```python
from build123d import *

# Parameters (mm, degrees)
BOX001_W         = 2
BOX001_H         = 37
BOX001_DEPTH     = 2
BOX_W            = 2
BOX_H            = 37
BOX_DEPTH        = 2
CIRCLE_R         = 1.75
EXTRUDE_DEPTH    = 2
CIRCLE001_R      = 1.75
EXTRUDE001_DEPTH = 2
CIRCLE002_R      = 1.75
EXTRUDE002_DEPTH = 2
CIRCLE003_R      = 1.75
EXTRUDE003_DEPTH = 2
RECTANGLE_W      = 43
RECTANGLE_H      = 43
EXTRUDE004_DEPTH = 2
FILLET_R         = 3
FILLET001_R      = 0.5
CHAMFER_SIZE     = 0.5
CHAMFER001_SIZE  = 0.5


with BuildPart() as cube001:
    # Box001 → Box001 (new body)
    with BuildSketch(Plane(origin=(30.5, 3, 0), x_dir=(1, 0, 0), z_dir=(0, 0, 1))):
        with Locations((1, 18.5)):
            Rectangle(BOX001_W, BOX001_H)
    extrude(amount=BOX001_DEPTH)


with BuildPart() as cube:
    # Box → Box (new body)
    with BuildSketch(Plane(origin=(10.5, 3, 0), x_dir=(1, 0, 0), z_dir=(0, 0, 1))):
        with Locations((1, 18.5)):
            Rectangle(BOX_W, BOX_H)
    extrude(amount=BOX_DEPTH)


with BuildPart() as extrude_body:
    # Circle → Extrude (new body)
    with BuildSketch(Plane(origin=(36.75, 6.25, 0), x_dir=(1, 0, 0), z_dir=(0, 0, 1))):
        Circle(CIRCLE_R)
    extrude(amount=EXTRUDE_DEPTH)


with BuildPart() as extrude001:
    # Circle001 → Extrude001 (new body)
    with BuildSketch(Plane(origin=(36.75, 36.75, 0), x_dir=(1, 0, 0), z_dir=(0, 0, 1))):
        Circle(CIRCLE001_R)
    extrude(amount=EXTRUDE001_DEPTH)


with BuildPart() as extrude002:
    # Circle002 → Extrude002 (new body)
    with BuildSketch(Plane(origin=(6.25, 6.25, 0), x_dir=(1, 0, 0), z_dir=(0, 0, 1))):
        Circle(CIRCLE002_R)
    extrude(amount=EXTRUDE002_DEPTH)


with BuildPart() as extrude003:
    # Circle003 → Extrude003 (new body)
    with BuildSketch(Plane(origin=(6.25, 36.75, 0), x_dir=(1, 0, 0), z_dir=(0, 0, 1))):
        Circle(CIRCLE003_R)
    extrude(amount=EXTRUDE003_DEPTH)


with BuildPart() as chamfer001:
    # Rectangle → Extrude004 (new body)
    with BuildSketch(Plane.XY):
        with Locations((21.5, 21.5)):
            Rectangle(RECTANGLE_W, RECTANGLE_H)
    extrude(amount=EXTRUDE004_DEPTH)

    # Cut: cut Extrude003
    add(extrude003.part, mode=Mode.SUBTRACT)

    # Cut001: cut Extrude002
    add(extrude002.part, mode=Mode.SUBTRACT)

    # Cut002: cut Extrude001
    add(extrude001.part, mode=Mode.SUBTRACT)

    # Cut003: cut Extrude body
    add(extrude_body.part, mode=Mode.SUBTRACT)

    # Cut004: cut Cube
    add(cube.part, mode=Mode.SUBTRACT)

    # Cut005: cut Cube001
    add(cube001.part, mode=Mode.SUBTRACT)

    # Fillet
    fillet_edges = [chamfer001.edges().sort_by_distance(p)[0] for p in [
        (0, 0, 1),
        (43, 0, 1),
        (0, 43, 1),
        (43, 43, 1),
    ]]
    fillet(fillet_edges, radius=FILLET_R)

    # Fillet001
    fillet001_edges = [chamfer001.edges().sort_by_distance(p)[0] for p in [
        (10.5, 3, 1),
        (10.5, 40, 1),
        (12.5, 40, 1),
        (12.5, 3, 1),
        (30.5, 3, 1),
        (30.5, 40, 1),
        (32.5, 3, 1),
        (32.5, 40, 1),
    ]]
    fillet(fillet001_edges, radius=FILLET001_R)

    # Chamfer
    chamfer_edges = [chamfer001.edges().sort_by_distance(p)[0] for p in [
        (10.5, 21.5, 2),
        (10.646447, 3.146447, 2),
        (10.646447, 39.853553, 2),
        (11.5, 3, 2),
        (11.5, 40, 2),
        (12.353553, 3.146447, 2),
        (12.353553, 39.853553, 2),
        (12.5, 21.5, 2),
        (35, 36.75, 2),
        (35, 6.25, 2),
        (4.5, 6.25, 2),
        (4.5, 36.75, 2),
        (30.5, 21.5, 2),
        (30.646447, 3.146447, 2),
        (30.646447, 39.853553, 2),
        (31.5, 3, 2),
        (31.5, 40, 2),
        (32.353553, 3.146447, 2),
        (32.353553, 39.853553, 2),
        (32.5, 21.5, 2),
    ]]
    chamfer(chamfer_edges, length=CHAMFER_SIZE)

    # Chamfer001
    chamfer001_edges = [chamfer001.edges().sort_by_distance(p)[0] for p in [
        (10.5, 21.5, 0),
        (10.646447, 3.146447, 0),
        (10.646447, 39.853553, 0),
        (11.5, 3, 0),
        (11.5, 40, 0),
        (12.353553, 3.146447, 0),
        (12.353553, 39.853553, 0),
        (12.5, 21.5, 0),
        (35, 36.75, 0),
        (35, 6.25, 0),
        (4.5, 6.25, 0),
        (4.5, 36.75, 0),
        (30.5, 21.5, 0),
        (30.646447, 3.146447, 0),
        (30.646447, 39.853553, 0),
        (31.5, 3, 0),
        (31.5, 40, 0),
        (32.353553, 3.146447, 0),
        (32.353553, 39.853553, 0),
        (32.5, 21.5, 0),
    ]]
    chamfer(chamfer001_edges, length=CHAMFER001_SIZE)


solid = chamfer001.part
```
Could you check a few things on this model? Use its own coordinates, in mm. A direction names the side the tool comes from. Give positions to 0.01 mm unless a question says otherwise; leave off trailing zeros. Loops run counter-clockwise (first coordinate to the right, second up) from the corner with the lowest first, then second, coordinate; pieces in that order, holes last. Notation, with made-up numbers: (87, 41.25) -> (118, 41.25) arc R10 cw to (118, 60.25) -> close; hole circle Ø2 at (-36.75, -13.75). An arc over 180 degrees is marked (long way). Put each result on its own line as item: value.
(1) Imagine slicing it at A-A on y = 9.5. Write out the boundary of the cut face in (x, z).
Computed:
outline: (0, 0) -> (10, 0) -> (10.5, 0.5) -> (10.5, 1.5) -> (10, 2) -> (0, 2) -> close; (12.5, 0.5) -> (13, 0) -> (30, 0) -> (30.5, 0.5) -> (30.5, 1.5) -> (30, 2) -> (13, 2) -> (12.5, 1.5) -> close; (32.5, 0.5) -> (33, 0) -> (43, 0) -> (43, 2) -> (33, 2) -> (32.5, 1.5) -> close
(2) For faces 5 (the face through (10.517, 3.006, 0.309)), 6 (the face through (10.5, 39.99, 1.7)), 7 (the face through (21, 0, 1)), 8 (the face through (32.5, 21, 1)), which set-ups out of +Z, -Z, +X, -X, +Y, -Y let a thin tool reach every point of the face, with its end or its side?
Computed:
face 5: -Z
face 6: +Z
face 7: +Z, -Z, +X, -X, -Y
face 8: +Z, -Z
(3) Thinking about a two-plate mould opening in Y: for faces 1 (the face through (21, 22, 2)), 2 (the face through (5.87, 4.54, 0.99)), 3 (the face through (32.49, 40, 1.7)), 4 (the face through (0.86, 42.1, 1.01)), which applies, pulls with the +Y half, pulls with the -Y half, needs draft (parallel to the pull), parting line crosses it, or undercut?
Computed:
face 1: needs draft
face 2: undercut
face 3: undercut
face 4: pulls with the +Y half
(4) Imagine slicing it at B-B on x = 36.75. Write out the boundary of the cut face in (y, z), plus the area to 3 significant figures.
Computed:
outline: (0, 0) -> (4, 0) -> (4.5, 0.5) -> (4.5, 1.5) -> (4, 2) -> (0, 2) -> close; (8, 0.5) -> (8.5, 0) -> (34.5, 0) -> (35, 0.5) -> (35, 1.5) -> (34.5, 2) -> (8.5, 2) -> (8, 1.5) -> close; (38.5, 0.5) -> (39, 0) -> (43, 0) -> (43, 2) -> (39, 2) -> (38.5, 1.5) -> close
area: 71.0 mm^2
(5) Please list where these lines run through material, in increasing order: probe 1 along Y at (x, z) = (36.75, 0.85); probe 2 along X at (y, z) = (17.5, 0.9); probe 3 along X at (y, z) = (25.5, 1.75). Write a range as [from, to].
Computed:
probe 1: [0, 4.5], [8, 35], [38.5, 43]
probe 2: [0, 10.5], [12.5, 30.5], [32.5, 43]
probe 3: [0, 10.25], [12.75, 30.25], [32.75, 43]
(6) Imagine slicing it at C-C on z = 0.9. Write out the boundary of the cut face in (x, y).
Computed:
outline: (0, 3) arc R3 ccw to (3, 0) -> (40, 0) arc R3 ccw to (43, 3) -> (43, 40) arc R3 ccw to (40, 43) -> (3, 43) arc R3 ccw to (0, 40) -> close; hole circle Ø3.5 at (6.25, 6.25); hole circle Ø3.5 at (6.25, 36.75); hole (10.5, 3.5) arc R0.5 ccw to (11, 3) -> (12, 3) arc R0.5 ccw to (12.5, 3.5) -> (12.5, 39.5) arc R0.5 ccw to (12, 40) -> (11, 40) arc R0.5 ccw to (10.5, 39.5) -> close; hole (30.5, 3.5) arc R0.5 ccw to (31, 3) -> (32, 3) arc R0.5 ccw to (32.5, 3.5) -> (32.5, 39.5) arc R0.5 ccw to (32, 40) -> (31, 40) arc R0.5 ccw to (30.5, 39.5) -> close; hole circle Ø3.5 at (36.75, 6.25); hole circle Ø3.5 at (36.75, 36.75)
